```python
from build123d import *

# Parameters (mm, degrees)
BOSS_EXTRUDE3_DEPTH   = 15.38
BOSS_EXTRUDE3_2_DEPTH = 15.38
BOSS_EXTRUDE3_3_DEPTH = 15.38
BOSS_EXTRUDE3_4_DEPTH = 15.38
BOSS_EXTRUDE3_5_DEPTH = 15.38
BOSS_EXTRUDE3_6_DEPTH = 15.38
SKETCH1_7_R           = 2
BOSS_EXTRUDE5_DEPTH   = 3
SKETCH1_8_R           = 2
SKETCH1_8_R_2         = 1
BOSS_EXTRUDE6_DEPTH   = 5


with BuildPart() as part:
    # Sketch1 → Boss-Extrude3 (new body)
    with BuildSketch(Plane(origin=(0, 0, 0), x_dir=(1, 0, 0), z_dir=(0, 1, 0))):
        Polygon((-128.783493648, 21.267304845), (-119.896742302, 5.875), (-118.536270399, 5.875), (-109.649519053, 21.267304845), align=None)
        Polygon((-113.979646072, 18.767304845), (-119.216506351, 9.69679677), (-124.453366629, 18.767304845), align=None, mode=Mode.SUBTRACT)
    extrude(amount=BOSS_EXTRUDE3_DEPTH)



with BuildPart() as body_2:
    # Sketch1 → Boss-Extrude3 2 (new body)
    with BuildSketch(Plane(origin=(0, 0, 0), x_dir=(1, 0, 0), z_dir=(0, 1, 0))):
        Polygon((-108.360471904, 0), (-99.473720558, 15.392304845), (-89.906733261, -1.17820323), (-107.680235952, -1.17820323), align=None)
        Polygon((-99.473720558, 10.392304845), (-94.23686028, 1.32179677), (-104.710580837, 1.32179677), align=None, mode=Mode.SUBTRACT)
    extrude(amount=BOSS_EXTRUDE3_2_DEPTH)


with BuildPart() as body_3:
    # Sketch1 → Boss-Extrude3 3 (new body)
    with BuildSketch(Plane(origin=(0, 0, 0), x_dir=(1, 0, 0), z_dir=(0, 1, 0))):
        Polygon((-130.752776749, -1.17820323), (-148.526279441, -1.17820323), (-138.959292143, 15.392304845), (-130.072540797, 0), align=None)
        Polygon((-144.196152422, 1.32179677), (-138.959292143, 10.392304845), (-133.722431864, 1.32179677), align=None, mode=Mode.SUBTRACT)
    extrude(amount=BOSS_EXTRUDE3_3_DEPTH)


with BuildPart() as body_4:
    # Sketch1 → Boss-Extrude3 4 (new body)
    with BuildSketch(Plane(origin=(0, 0, 0), x_dir=(1, 0, 0), z_dir=(0, 1, 0))):
        Polygon((-138.959292143, -29.498711305), (-130.072540797, -14.106406459), (-130.752776749, -12.92820323), (-148.526279441, -12.92820323), align=None)
        Polygon((-144.196152422, -15.42820323), (-133.722431864, -15.42820323), (-138.959292143, -24.498711305), align=None, mode=Mode.SUBTRACT)
    extrude(amount=BOSS_EXTRUDE3_4_DEPTH)


with BuildPart() as body_5:
    # Sketch1 → Boss-Extrude3 5 (new body)
    with BuildSketch(Plane(origin=(0, 0, 0), x_dir=(1, 0, 0), z_dir=(0, 1, 0))):
        Polygon((-89.906733261, -12.92820323), (-107.680235952, -12.92820323), (-108.360471904, -14.106406459), (-99.473720558, -29.498711305), align=None)
        Polygon((-99.473720558, -24.498711305), (-104.710580837, -15.42820323), (-94.23686028, -15.42820323), align=None, mode=Mode.SUBTRACT)
    extrude(amount=BOSS_EXTRUDE3_5_DEPTH)


with BuildPart() as body_6:
    # Sketch1 → Boss-Extrude3 6 (new body)
    with BuildSketch(Plane(origin=(0, 0, 0), x_dir=(1, 0, 0), z_dir=(0, 1, 0))):
        Polygon((-118.536270399, -19.981406459), (-109.649519053, -35.373711305), (-128.783493648, -35.373711305), (-119.896742302, -19.981406459), align=None)
        Polygon((-113.979646072, -32.873711305), (-124.453366629, -32.873711305), (-119.216506351, -23.80320323), align=None, mode=Mode.SUBTRACT)
    extrude(amount=BOSS_EXTRUDE3_6_DEPTH)


with BuildPart() as part_1:
    add(part.part)

    add(body_2.part)  # Boss-Extrude5 merges body 2

    add(body_3.part)  # Boss-Extrude5 merges body 3

    add(body_4.part)  # Boss-Extrude5 merges body 4

    add(body_5.part)  # Boss-Extrude5 merges body 5

    add(body_6.part)  # Boss-Extrude5 merges body 6
    # Sketch1_7 → Boss-Extrude5 (add)
    with BuildSketch(Plane(origin=(0, 0, 0), x_dir=(1, 0, 0), z_dir=(0, 1, 0))):
        Polygon((-119.896742302, 5.875), (-128.783493648, 21.267304845), (-129.428017223, 10.633652423), (-138.959292143, 15.392304845), (-130.072540797, 0), (-130.752776749, -1.17820323), (-148.526279441, -1.17820323), (-139.639528095, -7.05320323), (-148.526279441, -12.92820323), (-130.752776749, -12.92820323), (-130.072540797, -14.106406459), (-138.959292143, -29.498711305), (-129.428017223, -24.740058882), (-128.783493648, -35.373711305), (-119.896742302, -19.981406459), (-118.536270399, -19.981406459), (-109.649519053, -35.373711305), (-109.004995479, -24.740058882), (-99.473720558, -29.498711305), (-108.360471904, -14.106406459), (-107.680235952, -12.92820323), (-89.906733261, -12.92820323), (-98.793484607, -7.05320323), (-89.906733261, -1.17820323), (-107.680235952, -1.17820323), (-108.360471904, 0), (-99.473720558, 15.392304845), (-109.004995479, 10.633652423), (-109.649519053, 21.267304845), (-118.536270399, 5.875), align=None)
        with Locations(Location((-119.216506351, -7.05320323, 0), (0, 0, 270))):
            Circle(SKETCH1_7_R, mode=Mode.SUBTRACT)
    extrude(amount=BOSS_EXTRUDE5_DEPTH)

    # Sketch1_8 → Boss-Extrude6 (add)
    with BuildSketch(Plane(origin=(0, 0, 0), x_dir=(1, 0, 0), z_dir=(0, 1, 0))):
        with Locations(Location((-119.216506351, -7.05320323, 0), (0, 0, 270))):
            Circle(SKETCH1_8_R)
        with Locations(Location((-119.216506351, -7.05320323, 0), (0, 0, 270))):
            Circle(SKETCH1_8_R_2, mode=Mode.SUBTRACT)
    extrude(amount=BOSS_EXTRUDE6_DEPTH)


solid = part_1.part
```
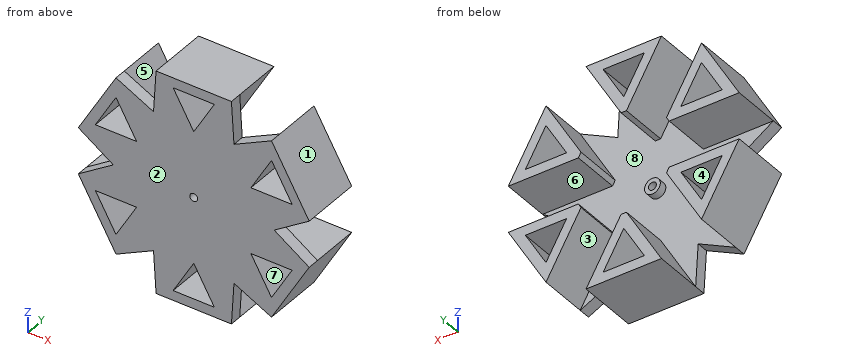
Source: CAD feature listing. Evaluate the final solid. Frame: model axes, mm. Face numbers are marked on the shaded views. A direction names the side the tool comes from. Round coordinates to 2 decimals unless told otherwise and drop trailing zeros. Loops run counter-clockwise (first coordinate to the right, second up) from the corner with the lowest first, then second, coordinate; pieces in that order, holes last. Notation, with made-up numbers: M -4,-36.5 L 55,-36.5 A24 ccw 55,0.5 Z; hole C -13,12 d9. An arc over 180 degrees is marked long. Use a Markdown table: item, result. Add a question column.
1. Pull-direction query (Z, two-part tool) for the marked faces 1, 2, 3 and 4; classes: +Z half, -Z half, draft (parallel to the pull), parting line (faces both ways), or undercut.
2. Contact query for flat-ended pins moving along their axis: pin 1 (3.5 mm diameter, centred on x = -139, y = 9.5, fed in from +Z); pin 2 (1 mm diameter, centred on y = 13, z = -4, fed in from -X); pin 3 (1.5 mm diameter, centred on y = 3, z = 18.5, fed in from +X). Output: stop coordinate, or through.
3. Cut plane C-C, the plane z = -14. Output: boundary loops of the cut face in (x, y).
4. Cut plane A-A, the plane y = 6.25. State how many separate pieces and enclosed holes the cut face has, and give its area (3 significant figures).
5. Ray query, line 1 along Z through (x, y) = (-134.5, 12) (3 decimals); line 2 along Z through (x, y) = (-124, 11); line 3 along X through (y, z) = (3.5, 23). Return the intervals inside material, ascending. Write a range as [from, to].
6. Set-up query: the marked faces 5, 6, 7 and 8. Return all of +Z, -Z, +X, -X, +Y, -Y with unobstructed straight access to the full face (end or side cutting, diameter ignored); none if empty.
7. Cut plane B-B, the plane x = -123. Output: boundary loops of the cut face in (y, z), and give its area (3 significant figures).
8. Cut plane D-D, the plane x = -143. Output: boundary loops of the cut face in (y, z).
Solution:
| question | item | result |
|---|---|---|
| 1 | face 1 | +Z half |
| 1 | face 2 | draft |
| 1 | face 3 | -Z half |
| 1 | face 4 | undercut |
| 2 | pin 1 | stops at z = 29.5 |
| 2 | pin 2 | stops at x = -145.83 |
| 2 | pin 3 | stops at x = -92.69 |
| 3 | outline | M -139.76,0 L -136.17,0 L -136.17,3 L -138.16,3 L -138.16,15.38 L -139.76,15.38 Z; M -129.22,0 L -121.7,0 L -121.7,15.38 L -124.59,15.38 L -124.59,3 L -129.22,3 Z; M -116.73,0 L -109.21,0 L -109.21,3 L -113.85,3 L -113.85,15.38 L -116.73,15.38 Z; M -102.26,0 L -98.67,0 L -98.67,15.38 L -100.28,15.38 L -100.28,3 L -102.26,3 Z |
| 4 | separate pieces | 6 |
| 4 | enclosed holes | 6 |
| 4 | area | 661 mm2 |
| 5 | line 1 | z = [-7.669, -2.669], [-1.322, 1.178], [12.928, 15.428], [16.775, 21.775] |
| 5 | line 2 | z = [-21.27, -18.77], [-17.98, -12.98], [27.09, 32.09], [32.87, 35.37] |
| 5 | line 3 | x = [-142.71, -139.82], [-138.09, -135.21], [-121.64, -116.79], [-103.23, -100.34], [-98.61, -95.72] |
| 6 | face 5 | +Z, +Y |
| 6 | face 6 | +X, -X, +Y |
| 6 | face 7 | +Y, -Y |
| 6 | face 8 | +Y |
| 7 | outline | M 0,-21.27 L 15.38,-21.27 L 15.38,-18.77 L 0,-18.77 Z; M 0,-16.25 L 15.38,-16.25 L 15.38,-11.25 L 3,-11.25 L 3,25.36 L 15.38,25.36 L 15.38,30.36 L 0,30.36 Z; M 0,32.87 L 15.38,32.87 L 15.38,35.37 L 0,35.37 Z |
| 7 | area | 341 mm2 |
| 8 | outline | M 0,-8.39 L 15.38,-8.39 L 15.38,-3.39 L 0,-3.39 Z; M 0,-1.32 L 15.38,-1.32 L 15.38,1.18 L 3,1.18 L 3,4.83 L 0,4.83 Z; M 0,9.27 L 3,9.27 L 3,12.93 L 15.38,12.93 L 15.38,15.43 L 0,15.43 Z; M 0,17.5 L 15.38,17.5 L 15.38,22.5 L 0,22.5 Z |
